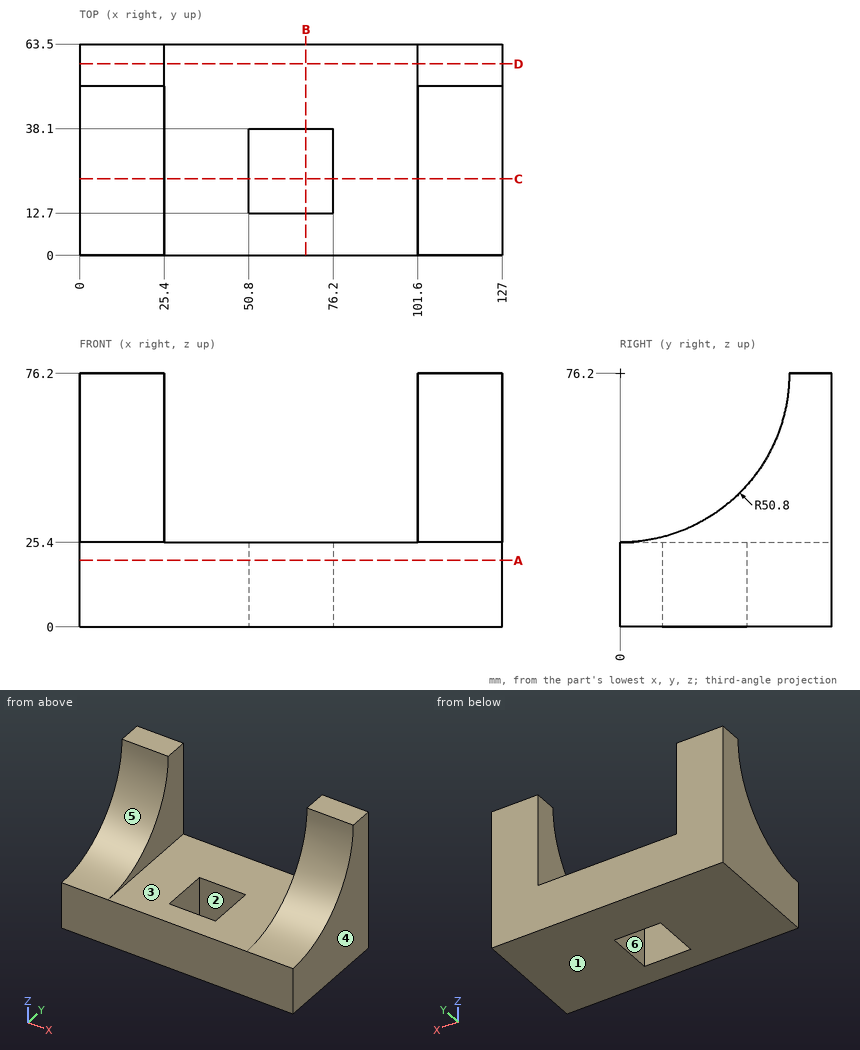
Study the drawing (mm; zero at the part's minimum x, y, z) and answer. A direction names the side the tool comes from. Coordinates: 2 decimals unless noted, no trailing zeros. Write each loop counter-clockwise with the first axis right and the second up, starting at its lowest first coordinate (ties: lowest second). Pieces come first, ordered by that corner, then holes. Notation, with made-up numbers: M 63.5,58.25 L 67.5,58.25 A16 cw 67.5,74.25 Z; hole C 34,-30 d9. An arc over 180 degrees is marked long. Use a Markdown table: item, result. Add a question column.
1. Straight lines are drawn through the part: line 1 along X through (y, z) = (17.5, 15); line 2 along X through (y, z) = (54, 66); line 3 along Z through (x, y) = (89, 16.5). For each, find the intervals that lie inside material, in ascending order. Write a range as [from, to].
2. Which of the six approach directions +Z, -Z, +X, -X, +Y, -Y give full straight-line access (tool end or side, diameter ignored) to the marked faces 1, 2 and 3?
3. Section D-D (y = 57.5) is taken. Give the vertices of the cut face in (x, z).
4. Section A-A (z = 20) is taken. Give the vertices of the cut face in (x, y), plus the area to 3 significant figures.
5. Section B-B (x = 68) is taken. Give the vertices of the cut face in (y, z).
6. Given P1, Ø19, axis at x = 79.5, y = 39.5, coming from the +Z side; P2, Ø5, axis at x = 100, y = 12, coming from the +Z side; P3, Ø3, axis at y = 20.5, z = 30, coming from the -X side; P4, Ø1.5, axis at x = 106.5, y = 10, coming from the +Z side, each flat-ended and moving along its own axis, determine where each tip first touches the part or whether it passes through.
7. Section C-C (y = 23) is taken. Give the vertices of the cut face in (x, z).
8. For a pull along X with two mould halves and no side action, classify the marked faces 4, 5 and 6 as +X half, -X half, draft (parallel to the pull), parting line (faces both ways), or undercut.
Data:
| question | item | result |
|---|---|---|
| 1 | line 1 | x = [0, 50.8], [76.2, 127] |
| 1 | line 2 | x = [0, 25.4], [101.6, 127] |
| 1 | line 3 | z = [0, 25.4] |
| 2 | face 1 | -Z, +X, -X, +Y, -Y |
| 2 | face 2 | +Z, -Z |
| 2 | face 3 | +Z, +Y, -Y |
| 3 | outline | M 0,0 L 127,0 L 127,76.2 L 101.6,76.2 L 101.6,25.4 L 25.4,25.4 L 25.4,76.2 L 0,76.2 Z |
| 4 | outline | M 0,0 L 127,0 L 127,63.5 L 0,63.5 Z; hole M 50.8,12.7 L 76.2,12.7 L 76.2,38.1 L 50.8,38.1 Z |
| 4 | area | 7,420 mm2 |
| 5 | outline | M 0,0 L 12.7,0 L 12.7,25.4 L 0,25.4 Z; M 38.1,0 L 63.5,0 L 63.5,25.4 L 38.1,25.4 Z |
| 6 | P1 | stops at z = 25.4 |
| 6 | P2 | stops at z = 27.34 |
| 6 | P3 | stops at x = 0 |
| 6 | P4 | stops at z = 26.55 |
| 7 | outline | M 0,0 L 50.8,0 L 50.8,25.4 L 25.4,25.4 L 25.4,30.9 L 0,30.9 Z; M 76.2,0 L 127,0 L 127,30.9 L 101.6,30.9 L 101.6,25.4 L 76.2,25.4 Z |
| 8 | face 4 | +X half |
| 8 | face 5 | draft |
| 8 | face 6 | undercut |
